Part model, mm, in its own coordinate system. A direction names the side the tool comes from. Round coordinates to 2 decimals unless told otherwise and drop trailing zeros. Write each loop counter-clockwise with the first axis right and the second up, starting at its lowest first coordinate (ties: lowest second). Pieces come first, ordered by that corner, then holes. Notation, with made-up numbers: (-3.5, 58.25) -> (17.5, 58.25) arc R29 cw to (17.5, 78.25) -> close; hole circle Ø3 at (29, -1). An arc over 180 degrees is marked (long way). Use CSV: the item, a comma, the result in double quotes. Start each with the question number.
(1) Two-plate mould, pull along X, no slides. Class faces 5 (the flat face through (-4.572, 28, 19)), 6 (the flat face through (28.684, 11.254, 19.492)), 7 (the flat face through (25.4, 6, 0)): released by +X, released by -X, zero draft, split by the parting line, or undercut.
(2) Drop flat-ended pins along their axis: pin 1 (1 mm diameter, centred on y = -7, z = 20.5, fed in from -X); pin 2 (5 mm diameter, centred on x = 15.5, y = -9.5, fed in from -Z); pin 3 (4 mm diameter, centred on x = 23, y = -19, fed in from -Z). Give the stop position or say it passes through.
(3) Saw through at B-B (y = 24). Count the separate pieces of the cut face and the enclosed holes in it, plus the area to 3 significant figures.
(4) Which spindle directions (+Z, -Z, +X, -X, +Y, -Y) get a long thin tool onto all of the face, cutting with end or side? Do faces 1 (the flat face through (-3, 16, 0)), 2 (the cylindrical face through (-1, 0.86, -3.88)), 3 (the flat face through (-3, 38, 38.446)), 4 (the flat face through (29, 16, 0)). Say none if no direction does.
(5) Probe line 1 (X direction, y = 19, z = 21.5); line 2 (X direction, y = 30.5, z = 14.5); line 3 (X direction, y = -6.5, z = 0.5). List the from-to ranges inside material, lowest first. Write a range as [from, to].
(6) Saw through at A-A (x = 3). Give the cut face in (y, z).
```python
from build123d import *

# Parameters (mm, degrees)
F0_R      = 32.113527
F1_DEPTH  = 25.4
F2_R      = 1.27
F3_R      = 1.27
F4_R      = 3.9751
F5_DEPTH  = 2.032
F7_R      = 3.9751
F8_DEPTH  = 2.032
F10_DEPTH = 2.54
F12_DEPTH = 2.54


with BuildPart() as f1:
    # F0 (on Right) → F1 (new body)
    with BuildSketch(Plane.YZ):
        Circle(F0_R)
    extrude(amount=F1_DEPTH)

    # F2
    f2_edges = [f1.edges().sort_by_distance(p)[0] for p in [
        (25.4, -32.113527, 0),
    ]]
    fillet(f2_edges, radius=F2_R)

    # F3
    f3_edges = [f1.edges().sort_by_distance(p)[0] for p in [
        (0, -32.113527, 0),
    ]]
    fillet(f3_edges, radius=F3_R)

    # F4 (on face) → F5 (join)
    with BuildSketch(Plane.YZ.offset(25.4)):
        Circle(F4_R)
    extrude(amount=F5_DEPTH)

    # F7 (on face) → F8 (join)
    with BuildSketch(Plane(origin=(0, 0, 0), x_dir=(0, -1, 0), z_dir=(-1, 0, 0))):
        Circle(F7_R)
    extrude(amount=F8_DEPTH)

    # F9 (on face) → F10 (join)
    with BuildSketch(Plane(origin=(-2.032, 0, 0), x_dir=(0, -1, 0), z_dir=(-1, 0, 0))):
        with BuildLine():
            ThreePointArc((-3.9751, 0), (-3.442538, 1.98755), (-1.98755, 3.442538))
            Line((-1.98755, 3.442538), (-22.197079, 38.446468))
            Line((-22.197079, 38.446468), (-54.258845, 38.446468))
            Line((-54.258845, 38.446468), (-32.061767, 0))
            Line((-32.061767, 0), (-3.9751, 0))
        make_face()
        with BuildLine():
            Line((-3.9751, 0), (0, 0))
            Line((0, 0), (-1.98755, 3.442538))
            ThreePointArc((-1.98755, 3.442538), (-3.442538, 1.98755), (-3.9751, 0))
        make_face()
    extrude(amount=F10_DEPTH)

    # F11 (on face) → F12 (join)
    with BuildSketch(Plane.YZ.offset(27.432)):
        Polygon((32.061767, 0), (54.258845, 38.446468), (22.197079, 38.446468), (0, 0), align=None)
    extrude(amount=F12_DEPTH)


solid = f1.part
```
Answers:
1,face 5,"released by -X"
1,face 6,"zero draft"
1,face 7,"undercut"
2,pin 1,"stops at x = 0"
2,pin 2,"stops at z = -31.34"
2,pin 3,"stops at z = -27.24"
3,separate pieces,"3"
3,enclosed holes,"0"
3,area,"1,280 mm²"
4,face 1,"-Z, -X, +Y, -Y"
4,face 2,"none"
4,face 3,"+Z, +X, -X, +Y, -Y"
4,face 4,"-Z, +X, +Y, -Y"
5,line 1,"x = [-4.57, -2.03], [0, 25.4], [27.43, 29.97]"
5,line 2,"x = [-4.57, -2.03], [27.43, 29.97]"
5,line 3,"x = [0, 25.4]"
6,outline,"circle Ø64.23 at (0, 0)"
